from build123d import *

# Parameters (mm, degrees)
SKETCH_1_W             = 153
SKETCH_1_H             = 45
SKETCH_1_R             = 10
SKETCH_1_R_2           = 4.25
EXTRUDE_1_DEPTH        = 5
SKETCH_6_R             = 12
CUT_EXTRUDE_1077_DEPTH = 8
SKETCH_9_W             = 90
SKETCH_9_H             = 115
EXTRUDE_2_DEPTH        = 10
HOLE_START             = -5
HOLE_WIZARD_2_DEPTH    = 5.7
HOLE_START_2           = 0.7
HOLE_WIZARD_2_2_DEPTH  = 4.3
CHAMFER_1_SIZE         = 5
FILLET_1_R             = 5
CHAMFER_2_SIZE         = 0.5
FILLET_2_R             = 10
SKETCH_13_R            = 20
CUT_EXTRUDE_1_DEPTH    = 10


# Read off the part's stored shape, not the designer's step: 打孔尺寸(%根据)内六角圆柱头螺钉的类型2
with BuildPart() as part:
    # 草图1 → 凸台-拉伸1 (new, symmetric)
    with BuildSketch(Plane(origin=(0, 0, 0), x_dir=(0, 0, -1), z_dir=(1, 0, 0))):
        with Locations((76.5, -22.5)):
            Rectangle(SKETCH_1_W, SKETCH_1_H)
        with Locations((28.5, -22.5)):
            Circle(SKETCH_1_R, mode=Mode.SUBTRACT)
        with Locations((85.5, -22.5)):
            Circle(SKETCH_1_R_2, mode=Mode.SUBTRACT)
        with Locations((130.5, -22.5)):
            Circle(SKETCH_1_R_2, mode=Mode.SUBTRACT)
    extrude(amount=EXTRUDE_1_DEPTH, both=True)

    # 草图6 → Cut-Extrude 1077 (cut)
    with BuildSketch(Plane.ZY.offset(-5)):
        with Locations((-28.5, -22.5)):
            Circle(SKETCH_6_R)
    extrude(amount=CUT_EXTRUDE_1077_DEPTH, mode=Mode.SUBTRACT)

    # 草图9 → 凸台-拉伸2 (add)
    with BuildSketch(Plane.ZY.offset(5)):
        with Locations((-45, 57.5)):
            Rectangle(SKETCH_9_W, SKETCH_9_H)
    extrude(amount=-EXTRUDE_2_DEPTH)

    # 打孔尺寸(%根据)内六角圆柱头螺钉的类型2 outline → 打孔尺寸(%根据)内六角圆柱头螺钉的类型2 (cut)
    with BuildSketch(Plane.YZ.offset(HOLE_START)):
        with BuildLine():
            ThreePointArc((55.758621971, -66.241378029), (50.758621971, -61.241378029), (45.758621971, -66.241378029))
            Line((45.758621971, -66.241378029), (45.758621971, -75.741378029))
            ThreePointArc((45.758621971, -75.741378029), (50.758621971, -80.741378029), (55.758621971, -75.741378029))
            Line((55.758621971, -75.741378029), (55.758621971, -66.241378029))
        make_face()
        with BuildLine():
            Line((55.758621971, -17.758621971), (55.758621971, -8.258621971))
            ThreePointArc((55.758621971, -8.258621971), (50.758621971, -3.258621971), (45.758621971, -8.258621971))
            Line((45.758621971, -8.258621971), (45.758621971, -17.758621971))
            ThreePointArc((45.758621971, -17.758621971), (50.758621971, -22.758621971), (55.758621971, -17.758621971))
        make_face()
        with BuildLine():
            ThreePointArc((113.741378029, -8.258621971), (108.741378029, -3.258621971), (103.741378029, -8.258621971))
            Line((103.741378029, -8.258621971), (103.741378029, -17.758621971))
            ThreePointArc((103.741378029, -17.758621971), (108.741378029, -22.758621971), (113.741378029, -17.758621971))
            Line((113.741378029, -17.758621971), (113.741378029, -8.258621971))
        make_face()
        with BuildLine():
            Line((113.741378029, -75.741378029), (113.741378029, -66.241378029))
            ThreePointArc((113.741378029, -66.241378029), (108.741378029, -61.241378029), (103.741378029, -66.241378029))
            Line((103.741378029, -66.241378029), (103.741378029, -75.741378029))
            ThreePointArc((103.741378029, -75.741378029), (108.741378029, -80.741378029), (113.741378029, -75.741378029))
        make_face()
    extrude(amount=HOLE_WIZARD_2_DEPTH, mode=Mode.SUBTRACT)

    # Hole Wizard 2 2 outline → Hole Wizard 2 2 (cut)
    with BuildSketch(Plane.YZ.offset(HOLE_START_2)):
        with BuildLine():
            ThreePointArc((53.508621971, -66.241378029), (50.758621971, -63.491378029), (48.008621971, -66.241378029))
            Line((48.008621971, -66.241378029), (48.008621971, -75.741378029))
            ThreePointArc((48.008621971, -75.741378029), (50.758621971, -78.491378029), (53.508621971, -75.741378029))
            Line((53.508621971, -75.741378029), (53.508621971, -66.241378029))
        make_face()
        with BuildLine():
            Line((53.508621971, -17.758621971), (53.508621971, -8.258621971))
            ThreePointArc((53.508621971, -8.258621971), (50.758621971, -5.508621971), (48.008621971, -8.258621971))
            Line((48.008621971, -8.258621971), (48.008621971, -17.758621971))
            ThreePointArc((48.008621971, -17.758621971), (50.758621971, -20.508621971), (53.508621971, -17.758621971))
        make_face()
        with BuildLine():
            ThreePointArc((111.491378029, -8.258621971), (108.741378029, -5.508621971), (105.991378029, -8.258621971))
            Line((105.991378029, -8.258621971), (105.991378029, -17.758621971))
            ThreePointArc((105.991378029, -17.758621971), (108.741378029, -20.508621971), (111.491378029, -17.758621971))
            Line((111.491378029, -17.758621971), (111.491378029, -8.258621971))
        make_face()
        with BuildLine():
            Line((111.491378029, -75.741378029), (111.491378029, -66.241378029))
            ThreePointArc((111.491378029, -66.241378029), (108.741378029, -63.491378029), (105.991378029, -66.241378029))
            Line((105.991378029, -66.241378029), (105.991378029, -75.741378029))
            ThreePointArc((105.991378029, -75.741378029), (108.741378029, -78.491378029), (111.491378029, -75.741378029))
        make_face()
    extrude(amount=HOLE_WIZARD_2_2_DEPTH, mode=Mode.SUBTRACT)

    # 倒角1
    chamfer_1_edges = [part.edges().sort_by_distance(p)[0] for p in [
        (0, -45, -153),
        (0, 0, -153),
    ]]
    chamfer(chamfer_1_edges, length=CHAMFER_1_SIZE)

    # 圆角1
    fillet_1_edges = [part.edges().sort_by_distance(p)[0] for p in [
        (0, -45, 0),
        (0, 115, -90),
        (0, 115, 0),
    ]]
    fillet(fillet_1_edges, radius=FILLET_1_R)

    # 倒角2
    chamfer_2_edges = [part.edges().sort_by_distance(p)[0] for p in [
        (5, -22.5, -40.5),
    ]]
    chamfer(chamfer_2_edges, length=CHAMFER_2_SIZE)

    # 圆角2
    fillet_2_edges = [part.edges().sort_by_distance(p)[0] for p in [
        (0, 0, -90),
    ]]
    fillet(fillet_2_edges, radius=FILLET_2_R)

    # 草图13 → 切除-拉伸1 (cut)
    with BuildSketch(Plane.ZY.offset(5)):
        with Locations((-42, 64.75)):
            Circle(SKETCH_13_R)
    extrude(amount=-CUT_EXTRUDE_1_DEPTH, mode=Mode.SUBTRACT)


solid = part.part
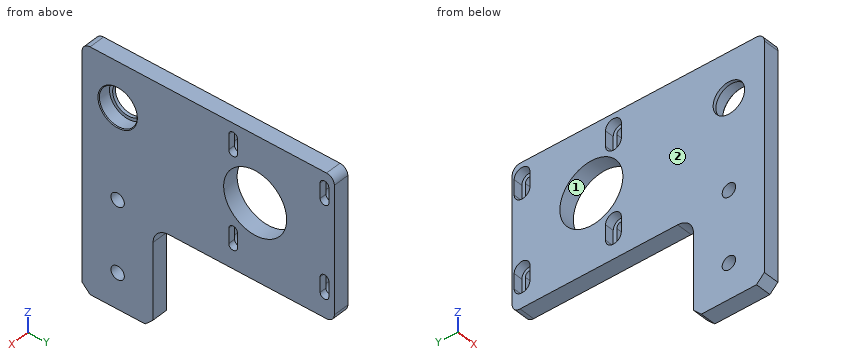
Could you check a few things on this model? Use its own coordinates, in mm. Face numbers are marked on the shaded views. Give positions to 0.01 mm unless a question says otherwise; leave off trailing zeros. Loops run counter-clockwise (first coordinate to the right, second up) from the corner with the lowest first, then second, coordinate; pieces in that order, holes last. Notation, with made-up numbers: (58.25, 29.5) -> (80.25, 29.5) arc R19 ccw to (80.25, 43.5) -> close; hole circle Ø8 at (5, 73). An arc over 180 degrees is marked (long way). Answer as CSV lines item,"result". Start each with the question number.
(1) I'm going to push flat-ended pins straight in: pin 1 Ø3 at (x, y) = (-1, 50.5) entering from -Z; pin 2 Ø11 at (y, z) = (52, -11) entering from -X. Where does each tip first touch, or does it pass through?
(2) I need wall thicknesses on probe 1 along Y at (x, z) = (-3.5, -31.5); probe 2 along Z at (x, y) = (0.5, 49.5); probe 3 along Y at (x, z) = (-3, -79). Which ranges of each line are inside material? Lowest first, please.
(3) If we section it at C-C on y = 64.75: Write out the boundary of the cut face in (x, z), then the cut area to 3 significant figures.
(4) If we section it at B-B on y = -22.5: Write out the boundary of the cut face in (x, z).
(5) If we section it at A-A on z = -130.5: Write out the boundary of the cut face in (x, y), then the cut area to 3 significant figures.
(6) If we section it at D-D on x = 2.5: Count the separate pieces of the cut face and the enclosed holes in it, then the cut area to 3 significant figures.
(7) We'd pull the mould along Y, two halves only. Please class the marked faces 1 and 2: released by +Y, released by -Y, zero draft, split by the parting line, or undercut.
Computed:
1,pin 1,"stops at z = -90"
1,pin 2,"stops at x = -5"
2,probe 1,"y = -45 to -32.04, -12.96 to 47.73, 81.77 to 115"
2,probe 2,"z = -90 to -80.58, -61.4 to -54.94, -29.06 to -22.6, -3.42 to 0"
2,probe 3,"y = -45 to 46.97, 54.55 to 104.95, 112.53 to 115"
3,outline,"(-5, -90) -> (5, -90) -> (5, -62) -> (-5, -62) -> close; (-5, -22) -> (5, -22) -> (5, 0) -> (-5, 0) -> close"
3,area,"500 mm2"
4,outline,"(-5, -153) -> (5, -153) -> (5, -134.75) -> (-5, -134.75) -> close; (-5, -126.25) -> (5, -126.25) -> (5, -89.75) -> (-5, -89.75) -> close; (-5, -81.25) -> (5, -81.25) -> (5, -41) -> (4.5, -40.5) -> (-3, -40.5) -> (-3, -38.5) -> (-5, -38.5) -> close; (-5, -18.5) -> (-3, -18.5) -> (-3, -16.5) -> (4.5, -16.5) -> (5, -16) -> (5, 0) -> (-5, 0) -> close"
5,outline,"(-5, -45) -> (5, -45) -> (5, -26.75) -> (-5, -26.75) -> close; (-5, -18.25) -> (5, -18.25) -> (5, 0) -> (-5, 0) -> close"
5,area,"365 mm2"
6,separate pieces,"1"
6,enclosed holes,"8"
6,area,"15,100 mm2"
7,face 1,"undercut"
7,face 2,"zero draft"
